Job drawing, mm, ordinate dimensions from the low corner. One solid piece. A direction names the side the tool comes from. Round coordinates to 2 decimals unless told otherwise and drop trailing zeros. Return JSON: item names as keys, results as strings. Group by question number.
Q1. Flat gauge pins, fed straight in: pin 1 (1.5 mm diameter, centred on y = 1, z = 1.5, fed in from -X); pin 2 (1 mm diameter, centred on x = 1, z = 3.5, fed in from +Y) (1 decimal). Where does each tip first touch, or does it go through?
Q2. Probe line 1 along Z through (x, y) = (1.9, 1.75); line 2 along Y through (x, z) = (4.45, 4.6) (1 decimal); line 3 along Y through (x, z) = (3.6, 2.2) (1 decimal). List the from-to ranges inside material, lowest first.
Q3. Which spindle directions (+Z, -Z, +X, -X, +Y, -Y) get a long thin tool onto all of the face, cutting with end or side? Do the marked faces 1, 2, 3 and 4. Say none if no direction does.
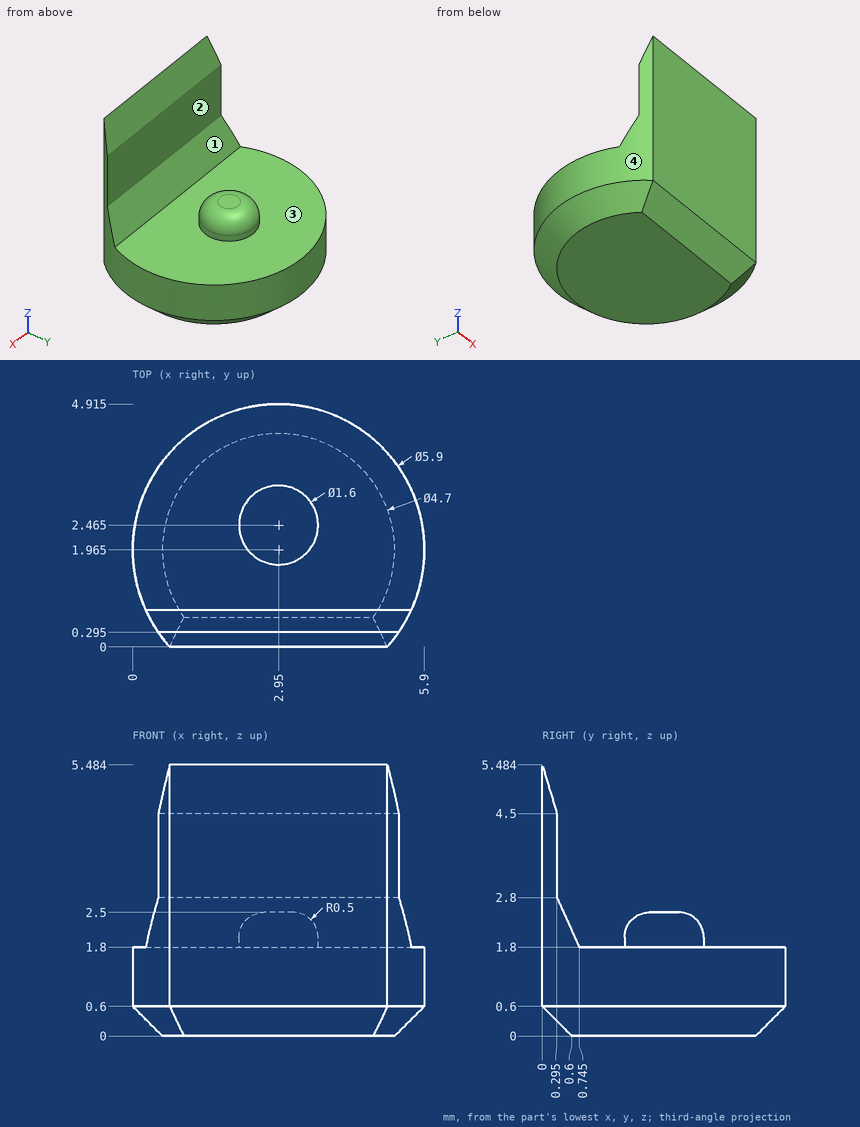
Solution:
{
 "1": {"pin 1": "stops at x = 0.01", "pin 2": "stops at y = 0.3"},
 "2": {"line 1": "z = 0 to 1.8", "line 2": "y = 0 to 0.3", "line 3": "y = 0 to 0.6, 2.1 to 2.9"},
 "3": {"face 1": "+Z, +X, -X", "face 2": "+Z, +X, -X, +Y", "face 3": "+Z", "face 4": "+Z, -Z"}
}
